Autodesk Fusion 360 part; units mm, degrees
sketch "Sketch1" plane through (0, 0, 0) normal (0, 1, 0) x (1, 0, 0)
  line L0 (0, 0) -> (30, 0)
  line L1 (30, 0) -> (30, -30)
  line L2 (30, -30) -> (0, -30)
  line L3 (0, -30) -> (0, 0)
  dimension "d1" = 30
extrude "Extrude1" add sketch "Sketch1" along normal blind 12.8
sketch "Sketch2" plane through (0, 12.8, 0) normal (0, 1, 0) x (-1, 0, 0)
  line L0 (0, 30) -> (-30, 30)
  line L1 (-30, 30) -> (-30, 0)
  line L2 (-30, 0) -> (0, 0)
  line L3 (0, 0) -> (0, 30)
  line L4 (0, 15) -> (-30, 15) construction
  line L5 (-15, 0) -> (-15, 30) construction
  circle A0 centre (-15, 15) radius 4.5
  line L6 (-3, 27) -> (-27, 27) construction
  line L7 (-27, 27) -> (-27, 3) construction
  line L8 (-27, 3) -> (-3, 3) construction
  line L9 (-3, 3) -> (-3, 27) construction
  line L10 (-3, 27) -> (-27, 3) construction
  line L11 (-27, 27) -> (-3, 3) construction
  point P0 (-15, 15)
  point P1 (-15, 15)
  point P2 (-27, 3)
  point P3 (-3, 3)
  point P4 (-3, 27)
  point P5 (-27, 27)
  dimension "d7" = 9
  dimension "d14" = 24
  dimension "d15" = 24
sketch "Sketch3" plane through (0, 0, 0) normal (0, -1, 0) x (1, 0, 0)
  line L0 (30, 30) -> (0, 30)
  line L1 (0, 30) -> (0, 0)
  line L2 (0, 0) -> (30, 0)
  line L3 (30, 0) -> (30, 30)
  circle A0 centre (15, 15) radius 11.075
  circle A1 centre (15, 15) radius 10.55
  dimension "d11" = 22.15
  dimension "d31" = 21.1
hole "Hole2" at (3, 12.8, 3) direction (0, -1, 0) diameter 3.3 end through all
hole "Hole3" at (27, 12.8, 3) direction (0, -1, 0) diameter 3.3 end through all
hole "Hole4" at (27, 12.8, 27) direction (0, -1, 0) diameter 3.3 end through all
hole "Hole5" at (3, 12.8, 27) direction (0, -1, 0) diameter 3.3 end through all
extrude "Extrude7" cut sketch "Sketch3" against normal blind 7 contours A0
extrude "Extrude8" cut sketch "Sketch3" against normal through all contours A1
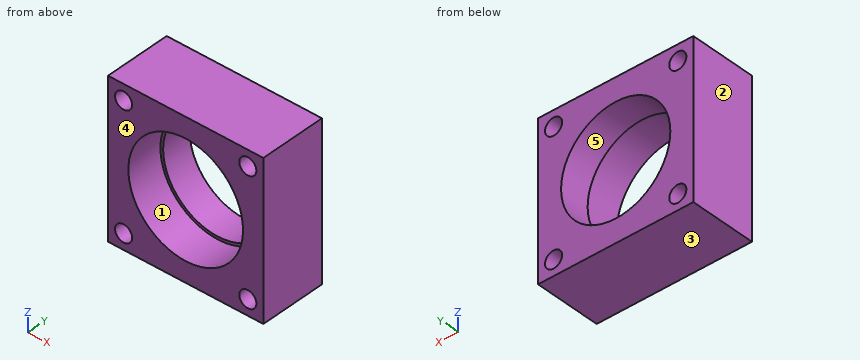
The model under review builds one solid part; all positions refer to its coordinate system, in mm. Face numbers are marked on the shaded views. A direction names the side the tool comes from. Give positions to 0.01 mm unless a question says otherwise; leave off trailing zeros. Order: outer loops, then holes, each group sorted by start corner. A loop starts at its lowest first (then second) coordinate and runs counter-clockwise, first axis right, second up. Notation, with made-up numbers: M -30,-7 L -23,-7 A25 ccw -23,28 Z; hole C -36.75,78.25 d11. An arc over 180 degrees is marked long. Use one line per item in the form item = value. Start each with the question number.
Item 1: We need section C-C on z = 3. Give the boundary of the cut face in (x, y).
Item 2: To check wall thickness, follow line 1 along X through (y, z) = (9.75, 3); line 2 along Z through (x, y) = (15, 8.25). State the ranges of each line that lie inside material, in increasing order. Write a range as from..to.
Item 3: We need section D-D on y = 5. Give the boundary of the cut face in (x, z) (3 decimals).
Item 4: Insertion check: pin 1 Ø8 at (x, z) = (10.5, 13) entering from +Y. The pin has a flat end and moves straight along its axis. Give the tip position at first contact, or say it passes through.
Item 5: For the marked faces 1 and 2, list the 3-axis set-ups (+Z, -Z, +X, -X, +Y, -Y) from which the entire face can be reached by the end or side of a thin tool; tool diameter is ignored.
Item 6: We need section A-A on x = 27. Give the boundary of the cut face in (y, z), plus the area to 3 significant figures.
Item 7: The part is to be moulded in two halves that separate along Z. For the marked faces 3, 4 and 5, say which applies: pulls with the +Z half, pulls with the -Z half, needs draft (parallel to the pull), parting line crosses it, or undercut.
Item 8: We need section B-B on x = 15. Give the boundary of the cut face in (y, z) (3 decimals), plus the area to 3 significant figures.
Completed:
q1.outline = M 0,0 L 1.35,0 L 1.35,12.8 L 0,12.8 Z; M 4.65,0 L 25.35,0 L 25.35,12.8 L 4.65,12.8 Z; M 28.65,0 L 30,0 L 30,12.8 L 28.65,12.8 Z
q2.line_1 = 0..1.35, 4.65..25.35, 28.65..30
q2.line_2 = 0..4.45, 25.55..30
q3.outline = M 0,0 L 30,0 L 30,30 L 0,30 Z; hole C 3,3 d3.3; hole C 3,27 d3.3; hole C 15,15 d22.15; hole C 27,3 d3.3; hole C 27,27 d3.3
q4.pin_1 = through
q5.face_1 = -Y
q5.face_2 = +Z, -Z, -X, +Y, -Y
q6.outline = M 0,0 L 12.8,0 L 12.8,1.35 L 0,1.35 Z; M 0,4.65 L 12.8,4.65 L 12.8,25.35 L 0,25.35 Z; M 0,28.65 L 12.8,28.65 L 12.8,30 L 0,30 Z
q6.area = 300 mm²
q7.face_3 = pulls with the -Z half
q7.face_4 = needs draft
q7.face_5 = undercut
q8.outline = M 0,0 L 12.8,0 L 12.8,4.45 L 7,4.45 L 7,3.925 L 0,3.925 Z; M 0,26.075 L 7,26.075 L 7,25.55 L 12.8,25.55 L 12.8,30 L 0,30 Z
q8.area = 107 mm²
